Could you check a few things on this model? Use its own coordinates, in mm. A direction names the side the tool comes from. Give positions to 0.01 mm unless a question says otherwise; leave off trailing zeros. Order: outer loops, then holes, each group sorted by start corner. A loop starts at its lowest first (then second) coordinate and runs counter-clockwise, first axis right, second up.
(1) Imagine slicing it at A-A, the plane x = 30. Write out the boundary of the cut face in (y, z), then the cut area to 3 significant figures.
(2) If I drill on probe 1 along Y at (x, z) = (30, 3.25); probe 2 along X at (y, z) = (-1, 47.5); probe 3 along Z at (x, y) = (26.5, 3), over which ranges is the centre line in solid material (lowest first)?
(3) Will these pins go through, and if not, where does the flat tip stop? pin 1 (4 mm diameter, centred on x = -10.5, y = 52.5, fed in from -Z); pin 2 (12 mm diameter, centred on x = 46, y = -9.5, fed in from +Z); pin 3 (1 mm diameter, centred on y = -37, z = 47.5, fed in from -X); pin 4 (20 mm diameter, centred on x = 31.5, y = 2, fed in from -Z).
(4) Imagine slicing it at B-B, the plane z = 32.5. Write out the boundary of the cut face in (x, y).
(5) Imagine slicing it at D-D, the plane x = 53.5. Write out the boundary of the cut face in (y, z), then the cut area to 3 significant figures.
(6) Imagine slicing it at C-C, the plane y = 0. Write out the boundary of the cut face in (x, z).
(7) If we mould it in two halves opening along Y, with no side actions, what happens to faces 1 (the flat face through (74, 1, 60)), 2 (the flat face through (1, -70, 30)), 3 (the flat face through (30, 0, 15))? For each: released by +Y, released by -Y, zero draft, split by the parting line, or undercut.
(8) On a 3-axis mill with a long thin cutter (end or side, diameter ignored), from which of +Z, -Z, +X, -X, +Y, -Y can I reach the whole of each face in a straight line? I mean faces 4 (the flat face through (9, 1, 25)), 5 (the cylindrical face through (10.924, 6.007, 7.395)), 6 (the flat face through (-50, -1, 23)). Say none if no direction works.
from build123d import *

# Parameters (mm, degrees)
EXTRUDE_1_DEPTH     = 60
SKETCH_2_W          = 120
SKETCH_2_H          = 94
CUT_EXTRUDE_1_DEPTH = 35
SKETCH_3_R          = 20
CUT_EXTRUDE_2_DEPTH = 15


with BuildPart() as part:
    # ｽｹｯﾁ1 → ﾎﾞｽ - 押し出し1 (new body)
    with BuildSketch(Plane.XY):
        with BuildLine():
            Line((-50, 70), (50, 70))
            ThreePointArc((50, 70), (120, 0), (50, -70))
            Line((50, -70), (-50, -70))
            Line((-50, -70), (-50, 70))
        make_face()
    extrude(amount=EXTRUDE_1_DEPTH)

    # ｽｹｯﾁ2 → ｶｯﾄ - 押し出し1 (cut)
    with BuildSketch(Plane.XY.offset(60)):
        with Locations((10, 0)):
            Rectangle(SKETCH_2_W, SKETCH_2_H)
    extrude(amount=-CUT_EXTRUDE_1_DEPTH, mode=Mode.SUBTRACT)

    # ｽｹｯﾁ3 → ｶｯﾄ - 押し出し2 (cut)
    with BuildSketch(Plane(origin=(0, 0, 0), x_dir=(-1, 0, 0), z_dir=(0, 0, -1))):
        with Locations((-30, 0)):
            Circle(SKETCH_3_R)
    extrude(amount=-CUT_EXTRUDE_2_DEPTH, mode=Mode.SUBTRACT)


solid = part.part
Answer block:
1. outline: (-70, 0) - (-20, 0) - (-20, 15) - (20, 15) - (20, 0) - (70, 0) - (70, 60) - (47, 60) - (47, 25) - (-47, 25) - (-47, 60) - (-70, 60) - close
1. area: 4,510 mm2
2. probe 1: y = -70 to -20, 20 to 70
2. probe 2: x = 70 to 119.99
2. probe 3: z = 15 to 25
3. pin 1: stops at z = 0
3. pin 2: stops at z = 25
3. pin 3: stops at x = 70
3. pin 4: stops at z = 15
4. outline: (-50, -70) - (50, -70) arc R70 ccw to (50, 70) - (-50, 70) - (-50, 47) - (70, 47) - (70, -47) - (-50, -47) - close
5. outline: (-69.91, 0) - (69.91, 0) - (69.91, 60) - (47, 60) - (47, 25) - (-47, 25) - (-47, 60) - (-69.91, 60) - close
5. area: 5,100 mm2
6. outline: (-50, 0) - (10, 0) - (10, 15) - (50, 15) - (50, 0) - (120, 0) - (120, 60) - (70, 60) - (70, 25) - (-50, 25) - close
7. face 1: zero draft
7. face 2: released by -Y
7. face 3: undercut
8. face 4: +Z, -X
8. face 5: -Z
8. face 6: +Z, -Z, -X, +Y, -Y
